Design review of the part built by this model. Coordinates are the model's own, in mm. Face numbers are marked on the shaded views. A direction names the side the tool comes from. Round coordinates to 2 decimals unless told otherwise and drop trailing zeros. Loops run counter-clockwise (first coordinate to the right, second up) from the corner with the lowest first, then second, coordinate; pieces in that order, holes last. Notation, with made-up numbers: M -28,-34.5 L 6,-34.5 A28 ccw 6,-0.5 Z; hole C 26.5,3.5 d10. An arc over 180 degrees is marked long. One line per item, written item: value. Start each with the question number.
Item 1: We need section D-D (y = 8.89). Write out the cut boundary in (x, z) (3 decimals).
Item 2: We need section A-A (z = 1.25). Write out the cut boundary in (x, y), then the cut area to 3 significant figures.
Item 3: We need section C-C (x = 10.16). Write out the cut boundary in (y, z) (3 decimals), then the cut area to 3 significant figures.
Item 4: We need section B-B (y = 1). Write out the cut boundary in (x, z) (3 decimals).
Item 5: For line 1 along Y through (x, z) = (0, 1.5); line 2 along Z through (x, y) = (-11.5, -3.25) (3 decimals); line 3 along Y through (x, z) = (2.5, 1.75), list the stretches that pass through material, from the lowest coordinate up.
Item 6: Mouldability with a two-part tool opening along X and no side actions: class the marked faces 1, 2 and 3 as released by +X, released by -X, zero draft, split by the parting line, or undercut.
Item 7: For the marked faces 4 and 5, list the 3-axis set-ups (+Z, -Z, +X, -X, +Y, -Y) from which the entire face can be reached by the end or side of a thin tool; tool diameter is ignored.
Item 8: Clearance check with flat-ended pins moving along their axes: pin 1 (1.5 mm diameter, centred on x = 9, z = 5, fed in from +Y); pin 2 (1.5 mm diameter, centred on y = -10, z = 5, fed in from +X); pin 3 (12.5 mm diameter, centred on x = -0.5, y = -4.5, fed in from +Z) (3 decimals). State where each tip first meets the part, or that it passes through.
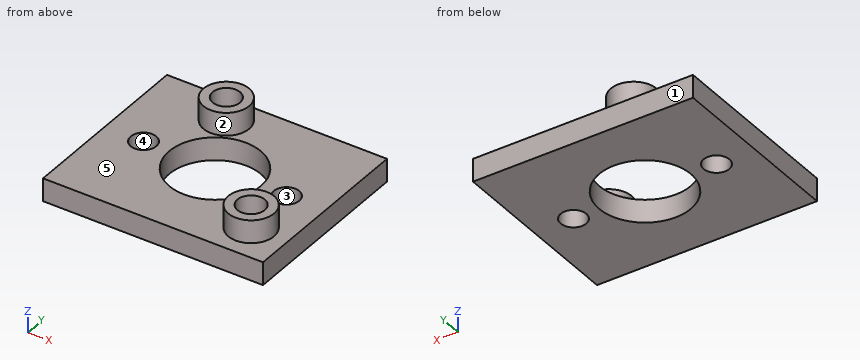
from build123d import *

# Parameters (mm, degrees)
SKETCH1_W           = 30.48
SKETCH1_H           = 25.4
SKETCH1_R           = 6.35
SKETCH1_R_2         = 1.778
BOSS_EXTRUDE1_DEPTH = 3.175
SKETCH2_R           = 3.175
SKETCH2_R_2         = 1.905
BOSS_EXTRUDE2_DEPTH = 3.175


with BuildPart() as part:
    # Sketch1 → Boss-Extrude1 (new body)
    with BuildSketch(Plane.XY):
        Rectangle(SKETCH1_W, SKETCH1_H)
        Circle(SKETCH1_R, mode=Mode.SUBTRACT)
        with Locations((-9.906, 0)):
            Circle(SKETCH1_R_2, mode=Mode.SUBTRACT)
        with Locations((9.906, 0)):
            Circle(SKETCH1_R_2, mode=Mode.SUBTRACT)
    extrude(amount=BOSS_EXTRUDE1_DEPTH)

    # Sketch2 → Boss-Extrude2 (add)
    with BuildSketch(Plane.XY.offset(3.175)):
        with Locations((-4.445, 8.89)):
            Circle(SKETCH2_R)
        with Locations((-4.445, 8.89)):
            Circle(SKETCH2_R_2, mode=Mode.SUBTRACT)
        with Locations((10.16, -7.62)):
            Circle(SKETCH2_R)
        with Locations((10.16, -7.62)):
            Circle(SKETCH2_R_2, mode=Mode.SUBTRACT)
    extrude(amount=BOSS_EXTRUDE2_DEPTH)


solid = part.part
A:
1. outline: M -15.24,0 L 15.24,0 L 15.24,3.175 L -1.27,3.175 L -1.27,6.35 L -2.54,6.35 L -2.54,3.175 L -6.35,3.175 L -6.35,6.35 L -7.62,6.35 L -7.62,3.175 L -15.24,3.175 Z
2. outline: M -15.24,-12.7 L 15.24,-12.7 L 15.24,12.7 L -15.24,12.7 Z; hole C -9.91,0 d3.56; hole C 0,0 d12.7; hole C 9.91,0 d3.56
2. area: 628 mm2
3. outline: M -12.7,0 L -1.76,0 L -1.76,3.175 L -4.445,3.175 L -4.445,6.35 L -5.715,6.35 L -5.715,3.175 L -9.525,3.175 L -9.525,6.35 L -10.795,6.35 L -10.795,3.175 L -12.7,3.175 Z; M 1.76,0 L 12.7,0 L 12.7,3.175 L 1.76,3.175 Z
3. area: 77.5 mm2
4. outline: M -15.24,0 L -11.376,0 L -11.376,3.175 L -15.24,3.175 Z; M -8.436,0 L -6.271,0 L -6.271,3.175 L -8.436,3.175 Z; M 6.271,0 L 8.436,0 L 8.436,3.175 L 6.271,3.175 Z; M 11.376,0 L 15.24,0 L 15.24,3.175 L 11.376,3.175 Z
5. line 1: -12.7 to -6.35, 6.35 to 12.7
5. line 2: 0 to 3.175
5. line 3: -12.7 to -5.84, 5.84 to 12.7
6. face 1: zero draft
6. face 2: split by the parting line
6. face 3: undercut
7. face 4: +Z, -Z
7. face 5: +Z
8. pin 1: y = -4.47
8. pin 2: x = 12.88
8. pin 3: z = 3.175
